from build123d import *

# Parameters (mm, degrees)
BOSS_EXTRUDE1_DEPTH     = 1.22
CUT_EXTRUDE2_DEPTH      = 246.803551555
CUT_EXTRUDE2_DEPTH_BACK = 246.803551555
SKETCH5_R               = 1.6
SKETCH6_R               = 27.5
SKETCH6_R_2             = 2
CUT_EXTRUDE3_DEPTH      = 42
CUT_EXTRUDE4_DEPTH      = 246.803551555
SKETCH8_R               = 5.75
CUT_EXTRUDE5_DEPTH      = 246.803551555


with BuildPart() as part:
    # Sketch1 → Boss-Extrude1 (new body)
    with BuildSketch(Plane(origin=(0, 0, 0), x_dir=(0, 0, -1), z_dir=(1, 0, 0))):
        with BuildLine():
            Line((-62.8, 9.646), (62.8, 9.646))
            ThreePointArc((62.8, 9.646), (63.428617928, 9.385617928), (63.689, 8.757))
            Line((63.689, 8.757), (63.689, -236.517))
            ThreePointArc((63.689, -236.517), (63.428617928, -237.145617928), (62.8, -237.406))
            Line((62.8, -237.406), (-62.8, -237.406))
            ThreePointArc((-62.8, -237.406), (-63.428617928, -237.145617928), (-63.689, -236.517))
            Line((-63.689, -236.517), (-63.689, 8.757))
            ThreePointArc((-63.689, 8.757), (-63.428617928, 9.385617928), (-62.8, 9.646))
        make_face()
    extrude(amount=BOSS_EXTRUDE1_DEPTH)

    # Sketch5 → Cut-Extrude2 (cut, two sides: drawn at the far end of the back side and taken through both)
    with BuildSketch(Plane(origin=(0, 0, 0), x_dir=(0, 0, -1), z_dir=(1, 0, 0)).offset(-CUT_EXTRUDE2_DEPTH_BACK)):
        with Locations((-47.5, -17.5)):
            Circle(SKETCH5_R)
        with Locations((0, -17.5)):
            Circle(SKETCH5_R)
        with Locations((47.5, -17.5)):
            Circle(SKETCH5_R)
        with Locations((-47.5, -107.5)):
            Circle(SKETCH5_R)
        with Locations((47.5, -107.5)):
            Circle(SKETCH5_R)
        with Locations((47.5, -120.26)):
            Circle(SKETCH5_R)
        with Locations((-47.5, -120.26)):
            Circle(SKETCH5_R)
        with Locations((47.5, -210.26)):
            Circle(SKETCH5_R)
        with Locations((0, -210.26)):
            Circle(SKETCH5_R)
        with Locations((-47.5, -210.26)):
            Circle(SKETCH5_R)
    extrude(amount=CUT_EXTRUDE2_DEPTH + CUT_EXTRUDE2_DEPTH_BACK, mode=Mode.SUBTRACT)

    # Sketch6 → Cut-Extrude3 (cut)
    with BuildSketch(Plane(origin=(0, 0, 0), x_dir=(0, 0, -1), z_dir=(1, 0, 0))):
        with Locations((0, -60)):
            Circle(SKETCH6_R)
        with Locations((0, -125)):
            Circle(SKETCH6_R)
        with Locations((24, -35)):
            Circle(SKETCH6_R_2)
        with Locations((-24, -35)):
            Circle(SKETCH6_R_2)
        with Locations((-24, -85)):
            Circle(SKETCH6_R_2)
        with Locations((24, -85)):
            Circle(SKETCH6_R_2)
        with Locations((24, -100)):
            Circle(SKETCH6_R_2)
        with Locations((-24, -100)):
            Circle(SKETCH6_R_2)
        with Locations((-24, -150)):
            Circle(SKETCH6_R_2)
        with Locations((24, -150)):
            Circle(SKETCH6_R_2)
    extrude(amount=CUT_EXTRUDE3_DEPTH, mode=Mode.SUBTRACT)

    # Sketch7 → Cut-Extrude4 (cut, through all)
    with BuildSketch(Plane(origin=(0, 0, 0), x_dir=(0, 0, -1), z_dir=(1, 0, 0))):
        with BuildLine():
            Line((-6.2, -189.6), (6.2, -189.6))
            ThreePointArc((6.2, -189.6), (6.376776695, -189.526776695), (6.45, -189.35))
            Line((6.45, -189.35), (6.45, -170.65))
            ThreePointArc((6.45, -170.65), (6.376776695, -170.473223305), (6.2, -170.4))
            Line((6.2, -170.4), (-6.2, -170.4))
            ThreePointArc((-6.2, -170.4), (-6.376776695, -170.473223305), (-6.45, -170.65))
            Line((-6.45, -170.65), (-6.45, -189.35))
            ThreePointArc((-6.45, -189.35), (-6.376776695, -189.526776695), (-6.2, -189.6))
        make_face()
    extrude(amount=CUT_EXTRUDE4_DEPTH, mode=Mode.SUBTRACT)

    # Sketch8 → Cut-Extrude5 (cut, through all)
    with BuildSketch(Plane(origin=(1.22, 0, 0), x_dir=(0, 0, -1), z_dir=(1, 0, 0))):
        with Locations((-23.75, -17.5)):
            Circle(SKETCH8_R)
        with Locations((23.75, -17.5)):
            Circle(SKETCH8_R)
    extrude(amount=-CUT_EXTRUDE5_DEPTH, mode=Mode.SUBTRACT)


solid = part.part
Source: CAD feature listing. Evaluate the final solid. Frame: model axes, mm. Round coordinates to 2 decimals unless told otherwise and drop trailing zeros. Order: outer loops, then holes, each group sorted by start corner. A loop starts at its lowest first (then second) coordinate and runs counter-clockwise, first axis right, second up. Notation, with made-up numbers: (33.5, 66.25) - (38.5, 66.25) arc R17 cw to (38.5, 98.25) - close; hole circle Ø2 at (-11, 46). An arc over 180 degrees is marked (long way). Use a Markdown table: item, result. Add a question column.
1. Section query A-A (y = -125). Return the cut outline in (x, z), then the cut area to 3 significant figures.
2. Section query C-C (y = -80). Return the cut outline in (x, z), then the cut area to 3 significant figures.
3. Section query B-B (x = 0.25). Give the number of separate pieces and of enclosed holes in the cut face, then the cut area to 3 significant figures.
4. First-contact query: pin 1 (6.5 mm diameter, centred on y = -150, z = 24, fed in from -X); pin 2 (1.9 mm diameter, centred on y = -107.5, z = -47.5, fed in from -X). Flat tips, straight axial feed; report the tip coordinate or a pass-through.
5. Mould query, pull axis Z, two halves, no side actions, for faces 1 (the cylindrical face through (0.601, -97.734, 3.58)), 2 (the flat face through (1.22, -112, 27)). Classes: +Z half, -Z half, draft (parallel to the pull), parting line (faces both ways), or undercut.
6. Line query: probe 1 along Z at (x, y) = (1.05, -210.26); probe 2 along Y at (x, z) = (0.95, 0); probe 3 along Y at (x, z) = (0.4, 47.5). Output: solid intervals per line, ascending.
Derived:
| question | item | result |
|---|---|---|
| 1 | outline | (0, -63.69) - (1.22, -63.69) - (1.22, -27.5) - (0, -27.5) - close; (0, 27.5) - (1.22, 27.5) - (1.22, 63.69) - (0, 63.69) - close |
| 1 | area | 88.3 mm2 |
| 2 | outline | (0, -63.69) - (1.22, -63.69) - (1.22, -18.87) - (0, -18.87) - close; (0, 18.87) - (1.22, 18.87) - (1.22, 63.69) - (0, 63.69) - close |
| 2 | area | 109 mm2 |
| 3 | separate pieces | 1 |
| 3 | enclosed holes | 23 |
| 3 | area | 26,100 mm2 |
| 4 | pin 1 | x = 0 |
| 4 | pin 2 | through |
| 5 | face 1 | undercut |
| 5 | face 2 | draft |
| 6 | probe 1 | -63.69 to -49.1, -45.9 to -1.6, 1.6 to 45.9, 49.1 to 63.69 |
| 6 | probe 2 | -237.41 to -211.86, -208.66 to -189.6, -170.4 to -152.5, -97.5 to -87.5, -32.5 to -19.1, -15.9 to 9.65 |
| 6 | probe 3 | -237.41 to -211.86, -208.66 to -121.86, -118.66 to -109.1, -105.9 to -19.1, -15.9 to 9.65 |
